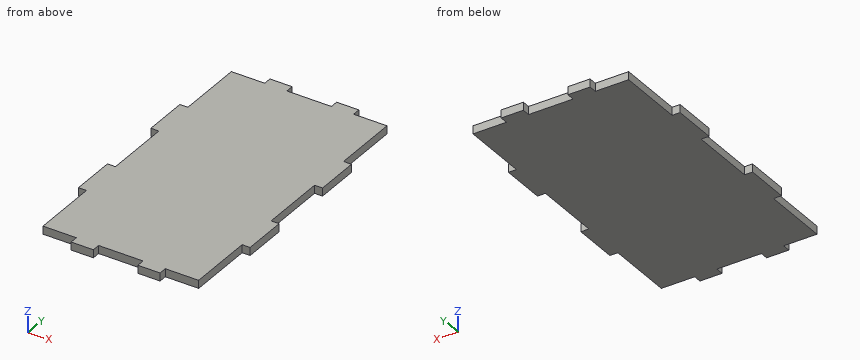
from build123d import *

# Parameters (mm, degrees)
SKETCH1_W           = 98.044
SKETCH1_H           = 174.244
BOSS_EXTRUDE1_DEPTH = 4.572
SKETCH2_W           = 23.622
SKETCH2_H           = 4.572
SKETCH2_W_2         = 25.4
CUT_EXTRUDE1_DEPTH  = 4.572
SKETCH3_W           = 4.572
SKETCH3_H           = 38.1
CUT_EXTRUDE2_DEPTH  = 4.572


with BuildPart() as part:
    # Sketch1 → Boss-Extrude1 (new body)
    with BuildSketch(Plane.XY):
        with Locations((49.022, 87.122)):
            Rectangle(SKETCH1_W, SKETCH1_H)
    extrude(amount=BOSS_EXTRUDE1_DEPTH)

    # Sketch2 → Cut-Extrude1 (cut)
    with BuildSketch(Plane.XY.offset(4.572)):
        with Locations((11.811, 2.286)):
            Rectangle(SKETCH2_W, SKETCH2_H)
        with Locations((49.022, 2.286)):
            Rectangle(SKETCH2_W_2, SKETCH2_H)
        with Locations((86.233, 2.286)):
            Rectangle(SKETCH2_W, SKETCH2_H)
        with Locations((11.811, 171.958)):
            Rectangle(SKETCH2_W, SKETCH2_H)
        with Locations((49.022, 171.958)):
            Rectangle(SKETCH2_W_2, SKETCH2_H)
        with Locations((86.233, 171.958)):
            Rectangle(SKETCH2_W, SKETCH2_H)
    extrude(amount=-CUT_EXTRUDE1_DEPTH, mode=Mode.SUBTRACT)

    # Sketch3 → Cut-Extrude2 (cut)
    with BuildSketch(Plane.XY.offset(4.572)):
        with Locations((2.286, 23.622)):
            Rectangle(SKETCH3_W, SKETCH3_H)
        with Locations((95.758, 23.622)):
            Rectangle(SKETCH3_W, SKETCH3_H)
        with Locations((2.286, 87.122)):
            Rectangle(SKETCH3_W, SKETCH3_H)
        with Locations((2.286, 150.622)):
            Rectangle(SKETCH3_W, SKETCH3_H)
        with Locations((95.758, 150.622)):
            Rectangle(SKETCH3_W, SKETCH3_H)
        with Locations((95.758, 87.122)):
            Rectangle(SKETCH3_W, SKETCH3_H)
    extrude(amount=-CUT_EXTRUDE2_DEPTH, mode=Mode.SUBTRACT)


solid = part.part
Read the model definition and answer for the solid it produces. Units are mm, in the model's axes. Coordinates: 2 decimals unless noted, no trailing zeros. Order: outer loops, then holes, each group sorted by start corner. A loop starts at its lowest first (then second) coordinate and runs counter-clockwise, first axis right, second up. Notation, with made-up numbers: M -34,-32.75 L -27,-32.75 A29 ccw -27,-11.75 Z; hole C 44,10.5 d7. An arc over 180 degrees is marked long. Put each result on its own line as item: value. Start each with the question number.
Item 1: Given pin 1 Ø1.4 at (y, z) = (3, 1.5) entering from -X; pin 2 Ø1 at (y, z) = (71, 1) entering from -X; pin 3 Ø1.4 at (x, z) = (80.5, 1.5) entering from +Y, each flat-ended and moving along its own axis, determine where each tip first touches the part or whether it passes through.
Item 2: Consider probe 1 along X at (y, z) = (12.5, 4.3); probe 2 along Y at (x, z) = (79.5, 3.5). Determine where each line is inside the solid, lowest interval first. Write a range as [from, to].
Item 3: Section A-A, the plane y = 99 is taken. Determine the outline of the cut face in (x, z), plus the area to 3 significant figures.
Item 4: Section B-B, the plane x = 59 is taken. Determine the outline of the cut face in (y, z), plus the area to 3 significant figures.
Computed:
1. pin 1: stops at x = 23.62
1. pin 2: stops at x = 4.57
1. pin 3: stops at y = 169.67
2. probe 1: x = [4.57, 93.47]
2. probe 2: y = [4.57, 169.67]
3. outline: M 4.57,0 L 93.47,0 L 93.47,4.57 L 4.57,4.57 Z
3. area: 406 mm2
4. outline: M 4.57,0 L 169.67,0 L 169.67,4.57 L 4.57,4.57 Z
4. area: 755 mm2
